Geometry: final body of the model. Coordinates: model frame, mm. Face numbers are marked on the shaded views. A direction names the side the tool comes from. Coordinates: 2 decimals unless noted, no trailing zeros. Write each loop counter-clockwise with the first axis right and the second up, starting at its lowest first coordinate (ties: lowest second). Pieces come first, ordered by that corner, then holes. Notation, with made-up numbers: M 1.25,-6 L 51.25,-6 A25 cw 51.25,14 Z; hole C -3,63 d1. An arc over 180 degrees is marked long. Write item = value, one per line. Start each with the question number.
Item 1: Section D-D on z = 18. Output: boundary loops of the cut face in (x, y).
Item 2: First-contact query: pin 1 Ø3 at (x, y) = (18, 10.5) entering from -Z; pin 2 Ø9 at (x, y) = (-10, 10) entering from +Z; pin 3 Ø3 at (y, z) = (16, 51.5) entering from +X. Flat tips, straight axial feed; report the tip coordinate or a pass-through.
Item 3: Ray query, L1, parallel to Z at x = 6.5, y = 5.5; L2, parallel to Y at x = 22, z = -25; L3, parallel to X at y = 7.5, z = -39. Return the intervals inside material, ascending. Write a range as [from, to].
Item 4: Section C-C on z = 40.5. Output: boundary loops of the cut face in (x, y).
Item 5: Section A-A on z = 0. Output: boundary loops of the cut face in (x, y), plus the area to 3 significant figures.
Item 6: Reachability of the marked faces 1 and 2 from +Z, -Z, +X, -X, +Y, -Y: full face, straight path, thin tool, end or side. Return the list, or none.
Item 7: Section B-B on x = 0. Output: boundary loops of the cut face in (y, z), plus the area to 3 significant figures.
Item 8: Pull-direction query (Z, two-part tool) for the marked faces 3, 4 and 5; classes: +Z half, -Z half, draft (parallel to the pull), parting line (faces both ways), or undercut.
from build123d import *

# Parameters (mm, degrees)
BOSS_EXTRUDE1_DEPTH = 20
FILLET1_R           = 10
SKETCH2_W           = 109
SKETCH2_H           = 77
CUT_EXTRUDE1_DEPTH  = 18.5
SKETCH4_R           = 8.25
SKETCH4_R_2         = 4.25
CUT_EXTRUDE2_DEPTH  = 10
SKETCH5_R           = 10
CUT_EXTRUDE3_DEPTH  = 10
SKETCH6_R           = 2.75
CUT_EXTRUDE4_DEPTH  = 30
CUT_EXTRUDE5_START  = -30
SKETCH7_R           = 2.75
CUT_EXTRUDE5_DEPTH  = 30
SKETCH8_R           = 5
CUT_EXTRUDE6_DEPTH  = 6
CUT_EXTRUDE7_START  = -6
SKETCH9_R           = 5
CUT_EXTRUDE7_DEPTH  = 6
SKETCH10_R          = 2.75
CUT_EXTRUDE8_DEPTH  = 20
SKETCH11_R          = 5
CUT_EXTRUDE9_DEPTH  = 5


with BuildPart() as part:
    # Sketch1 → Boss-Extrude1 (new body)
    with BuildSketch(Plane(origin=(0, 0, 0), x_dir=(1, 0, 0), z_dir=(0, 1, 0))):
        with BuildLine():
            Line((-50, -65), (50, -65))
            ThreePointArc((50, -65), (82.006097334, 0), (50, 65))
            Line((50, 65), (-50, 65))
            ThreePointArc((-50, 65), (-82.006097334, 0), (-50, -65))
        make_face()
    extrude(amount=BOSS_EXTRUDE1_DEPTH)

    # Fillet1
    fillet1_edges = [part.edges().sort_by_distance(p)[0] for p in [
        (-50, 10, -65),
        (50, 10, -65),
        (50, 10, 65),
        (-50, 10, 65),
    ]]
    fillet(fillet1_edges, radius=FILLET1_R)

    # Sketch2 → Cut-Extrude1 (cut)
    with BuildSketch(Plane(origin=(0, 20, 0), x_dir=(1, 0, 0), z_dir=(0, 1, 0))):
        with Locations((-12, 0)):
            Rectangle(SKETCH2_W, SKETCH2_H)
    extrude(amount=-CUT_EXTRUDE1_DEPTH, mode=Mode.SUBTRACT)

    # Sketch4 → Cut-Extrude2 (cut)
    with BuildSketch(Plane.XZ):
        with Locations(Location((30.815, 53.373145635, 0), (0, 0, 270))):
            Circle(SKETCH4_R)
        with Locations(Location((30.815, -53.373145635, 0), (0, 0, 270))):
            Circle(SKETCH4_R)
        with Locations(Location((-61.63, 0, 0), (0, 0, 270))):
            Circle(SKETCH4_R_2)
    extrude(amount=-CUT_EXTRUDE2_DEPTH, mode=Mode.SUBTRACT)

    # Sketch5 → Cut-Extrude3 (cut)
    with BuildSketch(Plane(origin=(0, 1.5, 0), x_dir=(1, 0, 0), z_dir=(0, 1, 0))):
        with Locations(Location((0, 0, 0), (0, 0, 270))):
            Circle(SKETCH5_R)
    extrude(amount=-CUT_EXTRUDE3_DEPTH, mode=Mode.SUBTRACT)

    # Sketch6 → Cut-Extrude4 (cut)
    with BuildSketch(Plane.XY.offset(65)):
        with Locations((-36.474488199, 10)):
            Circle(SKETCH6_R)
        with Locations((-10.000511801, 10)):
            Circle(SKETCH6_R)
        with Locations((16.474488199, 10)):
            Circle(SKETCH6_R)
    extrude(amount=-CUT_EXTRUDE4_DEPTH, mode=Mode.SUBTRACT)

    # Sketch7 → Cut-Extrude5 (cut)
    with BuildSketch(Plane(origin=(0, 0, -65), x_dir=(-1, 0, 0), z_dir=(0, 0, -1)).offset(CUT_EXTRUDE5_START)):
        with Locations(Location((-16.474488199, 10, 0), (0, 0, 180))):
            Circle(SKETCH7_R)
        with Locations(Location((10.000511801, 10, 0), (0, 0, 180))):
            Circle(SKETCH7_R)
        with Locations(Location((36.474488199, 10, 0), (0, 0, 180))):
            Circle(SKETCH7_R)
    extrude(amount=CUT_EXTRUDE5_DEPTH, mode=Mode.SUBTRACT)

    # Sketch8 → Cut-Extrude6 (cut)
    with BuildSketch(Plane.XY.offset(65)):
        with Locations((-36.474488199, 10)):
            Circle(SKETCH8_R)
        with Locations((-10.000511801, 10)):
            Circle(SKETCH8_R)
        with Locations((16.474488199, 10)):
            Circle(SKETCH8_R)
    extrude(amount=-CUT_EXTRUDE6_DEPTH, mode=Mode.SUBTRACT)

    # Sketch9 → Cut-Extrude7 (cut)
    with BuildSketch(Plane(origin=(0, 0, -65), x_dir=(-1, 0, 0), z_dir=(0, 0, -1)).offset(CUT_EXTRUDE7_START)):
        with Locations(Location((-16.474488199, 10, 0), (0, 0, 180))):
            Circle(SKETCH9_R)
        with Locations(Location((10.000511801, 10, 0), (0, 0, 180))):
            Circle(SKETCH9_R)
        with Locations(Location((36.474488199, 10, 0), (0, 0, 180))):
            Circle(SKETCH9_R)
    extrude(amount=CUT_EXTRUDE7_DEPTH, mode=Mode.SUBTRACT)

    # Sketch10 → Cut-Extrude8 (cut)
    with BuildSketch(Plane.XZ.offset(-10)):
        with Locations(Location((30.815, 53.373145635, 0), (0, 0, 270))):
            Circle(SKETCH10_R)
        with Locations(Location((30.815, -53.373145635, 0), (0, 0, 270))):
            Circle(SKETCH10_R)
    extrude(amount=-CUT_EXTRUDE8_DEPTH, mode=Mode.SUBTRACT)

    # Sketch11 → Cut-Extrude9 (cut)
    with BuildSketch(Plane(origin=(0, 20, 0), x_dir=(1, 0, 0), z_dir=(0, 1, 0))):
        with Locations(Location((30.815, 53.373145635, 0), (0, 0, 270))):
            Circle(SKETCH11_R)
        with Locations(Location((30.815, -53.373145635, 0), (0, 0, 270))):
            Circle(SKETCH11_R)
    extrude(amount=-CUT_EXTRUDE9_DEPTH, mode=Mode.SUBTRACT)


solid = part.part
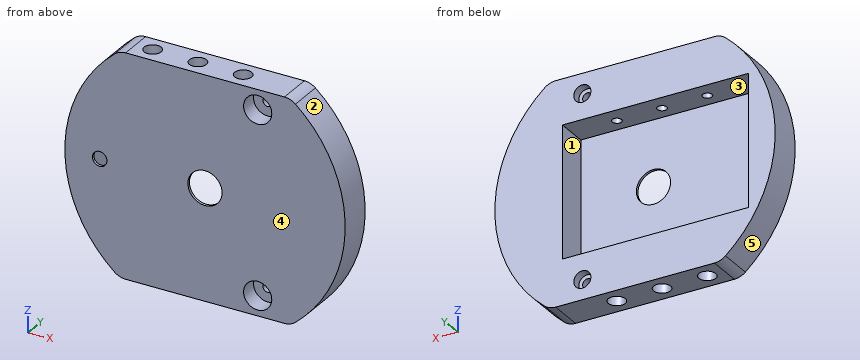
Responses:
q1.outline = M -80.01,0 L 80.01,0 L 80.01,20 L 42.5,20 L 42.5,1.5 L -66.5,1.5 L -66.5,20 L -80.01,20 Z
q2.pin_1 = -59
q2.pin_2 = 59
q2.pin_3 = 65
q3.L1 = [-65, -38.5], [38.5, 65]
q3.L2 = [0, 1.5]
q3.L3 = [-72.14, -37.62], [-35.33, -11.15], [-8.85, 15.33], [17.62, 72.14]
q4.outline = M -71.31,0 L 71.31,0 L 71.31,20 L -71.31,20 Z; hole C -36.47,10 d5.5; hole C -10,10 d5.5; hole C 16.47,10 d5.5
q5.outline = M -82.01,0 L -65.88,0 L -65.88,1.5 L -66.5,1.5 L -66.5,20 L -82.01,20 Z; M -57.38,0 L -10,0 L -10,1.5 L -57.38,1.5 Z; M 10,0 L 82.01,0 L 82.01,20 L 42.5,20 L 42.5,1.5 L 10,1.5 Z
q5.area = 1,220 mm²
q6.face_1 = +Y
q6.face_2 = +X, +Y, -Y
q7.outline = M 0,-65 L 20,-65 L 20,-38.5 L 1.5,-38.5 L 1.5,-10 L 0,-10 Z; M 0,10 L 1.5,10 L 1.5,38.5 L 20,38.5 L 20,65 L 0,65 Z
q7.area = 1,150 mm²
q8.face_3 = undercut
q8.face_4 = draft
q8.face_5 = parting line
